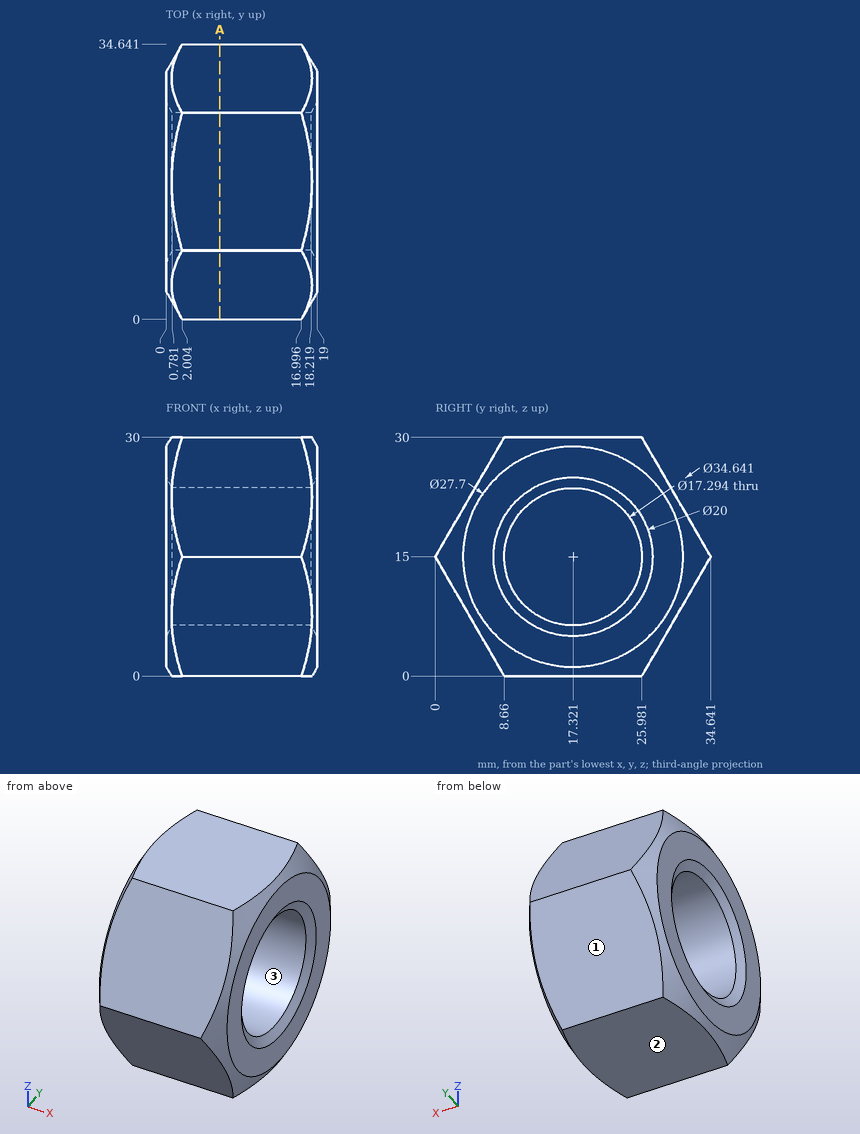
For this review, use the dimensioned drawing (mm, ordinates from the lowest corner) and the shaded views. Give positions to 0.01 mm unless a question says otherwise; leave off trailing zeros. Write each loop counter-clockwise with the first axis right and the second up, starting at its lowest first coordinate (ties: lowest second). Pieces come first, ordered by that corner, then holes. Notation, with made-up numbers: M -21,16 L 38,16 A12 cw 38,28 Z; hole C 71,-38 d10. An arc over 180 degrees is marked long. Answer as a JSON object with one key per item and string values. Group by question number.
1) We need section A-A (x = 6.75). Give the boundary of the cut face in (y, z) (1 decimal).
2) Mouldability with a two-part tool opening along Y and no side actions: class the marked faces 1, 2 and 3 as released by +Y, released by -Y, zero draft, split by the parting line, or undercut.
3) For line 1 along Y through (x, z) = (6, 15) (1 decimal); line 2 along Z through (x, y) = (10, 16) (1 decimal); line 3 along Z through (x, y) = (16, 13), list the stretches that pass through material, from the lowest coordinate up.
4) Clearance check with flat-ended pins moving along their axes: pin 1 Ø4 at (x, z) = (13.5, 8) entering from -Y; pin 2 Ø2 at (x, z) = (5, 26) entering from -Y; pin 3 Ø4 at (x, z) = (14.5, 8.5) entering from -Y. State where each tip first meets the part, or that it passes through.
Answer key:
{
 "1": {"outline": "M 0,15 L 8.7,0 L 26,0 L 34.6,15 L 26,30 L 8.7,30 Z; hole C 17.3,15 d17.3"},
 "2": {"face 1": "released by +Y", "face 2": "zero draft", "face 3": "undercut"},
 "3": {"line 1": "y = 0 to 8.7, 26 to 34.6", "line 2": "z = 0 to 6.5, 23.5 to 30", "line 3": "z = 0 to 7.51, 22.49 to 30"},
 "4": {"pin 1": "stops at y = 2.89", "pin 2": "stops at y = 5.77", "pin 3": "stops at y = 2.6"}
}
